CAD build for the part. Positions are in the model's coordinates, mm. A direction names the side the tool comes from. Round coordinates to 2 decimals unless told otherwise and drop trailing zeros. Loops run counter-clockwise (first coordinate to the right, second up) from the corner with the lowest first, then second, coordinate; pieces in that order, holes last.
from build123d import *

# Parameters (mm, degrees)
PAD021_DEPTH         = 3
SKETCH045_R          = 1.25
POCKET023_DEPTH      = 3.001
POCKET023_DEPTH_BACK = 0.001
POCKET024_DEPTH      = 1.8
PAD022_DEPTH         = 10
SKETCH048_W          = 8.6
SKETCH048_H          = 50.4
POCKET025_DEPTH      = 10
SKETCH049_W          = 2
SKETCH049_H          = 40
POCKET026_DEPTH      = 2
SKETCH050_W          = 1.2
SKETCH050_H          = 11.2
POCKET027_DEPTH      = 2
CHAMFER_SIZE         = 7
FILLET_R             = 2


with BuildPart() as part:
    # Sketch044 → Pad021 (new body)
    with BuildSketch(Plane.XY):
        with BuildLine():
            Line((-29.5, -64), (29.5, -64))
            ThreePointArc((29.5, -64), (31.267767, -63.267767), (32, -61.5))
            Line((32, -42.5), (32, -61.5))
            ThreePointArc((34.5, -40), (32.732233, -40.732233), (32, -42.5))
            Line((34.5, 12), (34.5, -40))
            ThreePointArc((32, 14.5), (32.732233, 12.732233), (34.5, 12))
            Line((32, 21.5), (32, 14.5))
            ThreePointArc((32, 21.5), (31.267767, 23.267767), (29.5, 24))
            Line((29.5, 24), (-34.5, 24))
            ThreePointArc((-34.5, 24), (-36.267767, 23.267767), (-37, 21.5))
            Line((-37, 21.5), (-37, -40))
            ThreePointArc((-37, -40), (-36.267767, -41.767767), (-34.5, -42.5))
            ThreePointArc((-32, -45), (-32.732233, -43.232233), (-34.5, -42.5))
            Line((-32, -45), (-32, -61.5))
            ThreePointArc((-32, -61.5), (-31.267767, -63.267767), (-29.5, -64))
        make_face()
    extrude(amount=-PAD021_DEPTH)

    # Sketch045 → Pocket023 (cut, two sides)
    with BuildSketch(Plane.XY) as pocket023_sk:
        with Locations((-34, 21)):
            Circle(SKETCH045_R)
        with Locations((27.5, 21)):
            Circle(SKETCH045_R)
        with Locations((27.5, -61)):
            Circle(SKETCH045_R)
        with Locations((-27.5, -61)):
            Circle(SKETCH045_R)
    extrude(amount=-POCKET023_DEPTH, mode=Mode.SUBTRACT)
    extrude(pocket023_sk.sketch, amount=POCKET023_DEPTH_BACK, mode=Mode.SUBTRACT)

    # Sketch046 (on Face5 of Pocket023) → Pocket024 (cut)
    with BuildSketch(Plane(origin=(0, 0, -3), x_dir=(1, 0, 0), z_dir=(0, 0, -1))):
        Polygon((-25.132864, 61), (-26.316432, 63.05), (-28.683568, 63.05), (-29.867136, 61), (-28.683568, 58.95), (-26.316432, 58.95), align=None)
        Polygon((29.867136, 61), (28.683568, 63.05), (26.316432, 63.05), (25.132864, 61), (26.316432, 58.95), (28.683568, 58.95), align=None)
        Polygon((-31.632864, -21), (-32.816432, -18.95), (-35.183568, -18.95), (-36.367136, -21), (-35.183568, -23.05), (-32.816432, -23.05), align=None)
        Polygon((29.867136, -21), (28.683568, -18.95), (26.316432, -18.95), (25.132864, -21), (26.316432, -23.05), (28.683568, -23.05), align=None)
    extrude(amount=-POCKET024_DEPTH, mode=Mode.SUBTRACT)

    # Sketch047 (on Face5 of Pocket024) → Pad022 (join)
    with BuildSketch(Plane(origin=(0, 0, -3), x_dir=(1, 0, 0), z_dir=(0, 0, -1))):
        with BuildLine():
            ThreePointArc((-34.5, 42.5), (-36.267767, 41.767767), (-37, 40))
            Line((-37, 40), (-37, -18.5))
            Line((-37, -18.5), (-29, -18.5))
            Line((-29, -18.5), (-29, -24))
            Line((-29, -24), (-22, -24))
            Line((-22, 45), (-22, -24))
            Line((-32, 45), (-22, 45))
            ThreePointArc((-34.5, 42.5), (-32.732233, 43.232233), (-32, 45))
        make_face()
    extrude(amount=PAD022_DEPTH)

    # Sketch048 → Pocket025 (cut)
    with BuildSketch(Plane.XY):
        with Locations((-32.7, -8)):
            Rectangle(SKETCH048_W, SKETCH048_H)
    extrude(amount=-POCKET025_DEPTH, mode=Mode.SUBTRACT)

    # Sketch049 (on Face50 of Pocket025) → Pocket026 (cut)
    with BuildSketch(Plane.XY.offset(-10)):
        with Locations((-34.5, -7.5)):
            Rectangle(SKETCH049_W, SKETCH049_H)
    extrude(amount=-POCKET026_DEPTH, mode=Mode.SUBTRACT)

    # Sketch050 → Pocket027 (cut)
    with BuildSketch(Plane.XY):
        with Locations((32.7, -4.9)):
            Rectangle(SKETCH050_W, SKETCH050_H)
    extrude(amount=-POCKET027_DEPTH, mode=Mode.SUBTRACT)

    # Chamfer
    chamfer_edges = [part.edges().sort_by_distance(p)[0] for p in [
        (-22, -10.5, -3),
    ]]
    chamfer(chamfer_edges, length=CHAMFER_SIZE)

    # Fillet
    fillet_edges = [part.edges().sort_by_distance(p)[0] for p in [
        (-22, -10.5, -13),
    ]]
    fillet(fillet_edges, radius=FILLET_R)


with BuildPart() as part_1:
    # Body006 placement: moved
    add(part.part.moved(Location((0, 0, -7))))


solid = part_1.part
Item 1: Cut at D-D (x = -17). List the corners of the cut face in (y, z), plus the area to 3 significant figures.
Verdict:
outline: (-64, -10) - (-45, -10) - (-45, -12) - (24, -12) - (24, -7) - (-64, -7) - close
area: 402 mm2
Item 2: Mould opens along Y. For faces 5 (the cylindrical face through (31.248, -63.287, -8.479)), 6 (the flat face through (-33, 18.5, -15)), 7 (the cylindrical face through (-27.66, -59.76, -7.59)) say: released by +Y, released by -Y, zero draft, split by the parting line, or undercut.
Verdict:
face 5: released by -Y
face 6: released by +Y
face 7: undercut
Item 3: Cut at C-C (z = -12.75). List the corners of the cut face in (x, y), plus the area to 3 significant figures.
Verdict:
outline: (-37, -40) arc R2.5 ccw to (-34.5, -42.5) arc R2.5 cw to (-32, -45) - (-17.75, -45) - (-17.75, 24) - (-29, 24) - (-29, 18.5) - (-37, 18.5) - (-37, 17.2) - (-28.4, 17.2) - (-28.4, -33.2) - (-37, -33.2) - close
area: 838 mm2
Item 4: 3-axis set-ups, long thin cutter, end or side, ignore diameter. For faces 1 (the flat face through (32, -52, -8)), 2 (the flat face through (-33, -8, -17)), 3 (the flat face through (-29.284, -59.989, -9.113)), 4 (the flat face through (-35, -27.5, -18)): which of +Z, -Z, +X, -X, +Y, -Y reach the whole face in a straight line?
Verdict:
face 1: +Z, -Z, +X, -Y
face 2: +Z, -X
face 3: -Z
face 4: +Z
Item 5: Cut at A-A (x = 27.5). List the corners of the cut face in (y, z).
Verdict:
outline: (-64, -10) - (-63.05, -10) - (-63.05, -8.2) - (-62.25, -8.2) - (-62.25, -7) - (-64, -7) - close; (-59.75, -8.2) - (-58.95, -8.2) - (-58.95, -10) - (18.95, -10) - (18.95, -8.2) - (19.75, -8.2) - (19.75, -7) - (-59.75, -7) - close; (22.25, -8.2) - (23.05, -8.2) - (23.05, -10) - (24, -10) - (24, -7) - (22.25, -7) - close
Item 6: Cut at B-B (y = -38). List the corners of the cut face in (x, z).
Verdict:
outline: (-37, -20) - (-24, -20) arc R2 ccw to (-22, -18) - (-22, -17) - (-15, -10) - (34.5, -10) - (34.5, -7) - (-37, -7) - close
Item 7: Flat gauge pins, fed straight in: P1, Ø1, axis at y = -10, z = -18, coming from the +X side; P2, Ø4, axis at x = -33.5, z = -17.5, coming from the +Y side; P3, Ø4.5, axis at x = -32, y = 21.5, coming from the -Z side; P4, Ø1.5, axis at x = -34, y = 21, coming from the +Z side. Where does each tip first touch, or does it go through?
Verdict:
P1: stops at x = -22
P2: stops at y = 18.5
P3: stops at z = -10
P4: passes through
Item 8: Wall check: L1, parallel to Y at x = 27.5, z = -7.9; L2, parallel to X at y = -25.5, z = -17.75; L3, parallel to Y at x = -34, z = -7.55. Give the ranges that are in metal, low to high.
Verdict:
L1: y = -64 to -62.25, -59.75 to 19.75, 22.25 to 24
L2: x = -37 to -35.5, -33.5 to -22
L3: y = -42.55 to -33.2, 17.2 to 19.75, 22.25 to 24
